Geometry: final body of the model. Coordinates: model frame, mm. A direction names the side the tool comes from. Give positions to 0.01 mm unless a question says otherwise; leave off trailing zeros. Loops run counter-clockwise (first coordinate to the right, second up) from the corner with the lowest first, then second, coordinate; pieces in that order, holes last. Notation, with made-up numbers: M 72,-27.5 L 130,-27.5 A15 cw 130,-9.5 Z; hole C 20.5,57 d10. An arc over 180 degrees is marked long. Put each result on its own line as item: value.
```python
from build123d import *

# Parameters (mm, degrees)
F3_R     = 0.8
F4_DEPTH = 1.204


with BuildPart() as f1:
    # F0 (on Front) → F1 (revolve)
    with BuildSketch(Plane.XZ):
        with BuildLine():
            Line((-4.65, 1.5564), (0, 1.5564))
            Line((0, 1.5564), (0, 16.5564))
            Line((0, 16.5564), (-2.7, 16.5564))
            ThreePointArc((-2.7, 16.5564), (-5.528427, 15.384827), (-6.7, 12.5564))
            Line((-6.7, 12.5564), (-6.7, -0.578493))
            Line((-6.7, -0.578493), (-5.455864, -0.578493))
            Line((-5.455864, -0.578493), (-5.455864, 0.040707))
            ThreePointArc((-5.455864, 0.040707), (-5.777928, 0.287836), (-5.9, 0.675))
            ThreePointArc((-5.9, 0.675), (-5.702297, 1.152297), (-5.225, 1.35))
            Line((-5.225, 1.35), (-4.65, 1.35))
            Line((-4.65, 1.35), (-4.65, 1.5564))
        make_face()
    revolve(axis=Axis((0, 0, 9.0564), (0, 0, -1)))

    # F3
    f3_edges = [f1.edges().sort_by_distance(p)[0] for p in [
        (6.7, 0, -0.578493),
    ]]
    fillet(f3_edges, radius=F3_R)

    # F2 (on face) → F4 (cut)
    with BuildSketch(Plane(origin=(0, 0, -0.578493), x_dir=(1, 0, 0), z_dir=(0, 0, -1))):
        Polygon((1, 10), (-1, 10), (-1, 0.57735), (-0.5, 0.866025), (0, 0), (0.5, 0.866025), (1, 0.57735), align=None)
        Polygon((-1, 0), (-1, 0.57735), (-9.160254, -4.133975), (-8.160254, -5.866025), (0, -1.154701), (-0.5, -0.866025), (0, 0), align=None)
        Polygon((9.160254, -4.133975), (1, 0.57735), (1, 0), (0, 0), (0.5, -0.866025), (0, -1.154701), (8.160254, -5.866025), align=None)
    extrude(amount=-F4_DEPTH, mode=Mode.SUBTRACT)


solid = f1.part
```
Item 1: Section A-A on z = 10.5. Output: boundary loops of the cut face in (x, y), then the cut area to 3 significant figures.
Output values:
outline: C 0,0 d13.4
area: 141 mm²
Item 2: Line query: probe 1 along Y at (x, z) = (0, 1.5); probe 2 along Z at (x, y) = (0.25, 1.5); probe 3 along X at (y, z) = (0.75, 0). Output: solid intervals per line, ascending. Write a range as [from, to].
Output values:
probe 1: [-6.7, -4.65], [4.65, 6.7]
probe 2: [1.56, 16.56]
probe 3: [-6.63, -5.4], [5.4, 6.63]
Item 3: Set-up query: faces 4 (the flat face through (4.683, 3.859, 0.015)), 5 (the cylindrical face through (-0.066, 5.455, -0.265)), 6 (the flat face through (-1, -6, 0)), 7 (the flat face through (-4.7, 3.87, 0.02)). Return all of +Z, -Z, +X, -X, +Y, -Y with unobstructed straight access to the full face (end or side cutting, diameter ignored); none if empty.
Output values:
face 4: -Z, +X
face 5: -Z
face 6: -Z, -Y
face 7: -Z, -X
Item 4: Pin query (flat end, axial travel): pin 1 Ø1 at (x, z) = (-3.5, 4) entering from +Y; pin 2 Ø0.6 at (y, z) = (-5.5, 0) entering from -X; pin 3 Ø5.5 at (x, y) = (0, 0) entering from -Z. Return the tip coordinate at first contact, or that it passes through.
Output values:
pin 1: y = 5.99
pin 2: x = -4.19
pin 3: z = 1.56
Item 5: Mould query, pull axis Y, two halves, no side actions, for faces 1 (the flat face through (1, -6, 0)), 2 (the flat face through (5.4, 3.1, 0.626)), 3 (the cylindrical face through (6.694, 0.295, 6.303)). Classes: pulls with the +Y half, pulls with the -Y half, needs draft (parallel to the pull), parting line crosses it, or undercut.
Output values:
face 1: needs draft
face 2: undercut
face 3: parting line crosses it
